from build123d import *

# Parameters (mm, degrees)
ESBO_O1_R                     = 8
RESSALTO_EXTRUS_O1_DEPTH      = 16
RESSALTO_EXTRUS_O3_START      = -2
ESBO_O3_R                     = 9.25
ESBO_O3_R_2                   = 8
RESSALTO_EXTRUS_O3_DEPTH      = 2
ESBO_O4_R                     = 7
CORTE_EXTRUS_O1_DEPTH         = 10
RESSALTO_EXTRUS_O2_DEPTH      = 4
RESSALTO_EXTRUS_O2_DEPTH_BACK = 16
ESBO_O2_R                     = 1.15
FILETE1_R                     = 1
PADR_O_LINEAR1_COUNT          = 11
PADR_O_LINEAR1_PITCH          = 0.5
CHANFRO1_SIZE                 = 0.2


with BuildPart() as part:
    # Esboço1 → Ressalto-extrusão1 (new body)
    with BuildSketch(Plane.XY):
        Circle(ESBO_O1_R)
    extrude(amount=RESSALTO_EXTRUS_O1_DEPTH)

    # Esboço3 → Ressalto-extrusão3 (add)
    with BuildSketch(Plane.XY.offset(7.5).offset(RESSALTO_EXTRUS_O3_START)):
        Circle(ESBO_O3_R)
        Circle(ESBO_O3_R_2, mode=Mode.SUBTRACT)
    extrude(amount=RESSALTO_EXTRUS_O3_DEPTH)

    # Esboço4 → Corte-extrusão1 (cut)
    with BuildSketch(Plane(origin=(0, 0, 0), x_dir=(-1, 0, 0), z_dir=(0, 0, -1))):
        Circle(ESBO_O4_R)
    extrude(amount=-CORTE_EXTRUS_O1_DEPTH, mode=Mode.SUBTRACT)

    # Esboço2 → Ressalto-extrusão2 (add, two sides: drawn at the far end of the back side and taken through both)
    with BuildSketch(Plane.XY.offset(16).offset(-RESSALTO_EXTRUS_O2_DEPTH_BACK)):
        with Locations((0, 4)):
            Circle(ESBO_O2_R)
        with Locations((3.708099244, -1.5)):
            Circle(ESBO_O2_R)
        with Locations((-3.708099244, -1.5)):
            Circle(ESBO_O2_R)
    extrude(amount=RESSALTO_EXTRUS_O2_DEPTH + RESSALTO_EXTRUS_O2_DEPTH_BACK)

    # Filete1
    filete1_edges = [part.edges().sort_by_distance(p)[0] for p in [
        (2.558099244, -1.5, 0),
        (-4.858099244, -1.5, 0),
        (-1.15, 4, 0),
    ]]
    fillet(filete1_edges, radius=FILETE1_R)

    # Esboço5 → Revolução1 (revolve)
    with BuildSketch(Plane(origin=(0, 0, 0), x_dir=(1, 0, 0), z_dir=(0, 1, 0)), mode=Mode.PRIVATE) as revolu_o1_sk:
        Polygon((8, 0), (8.433012702, -0.25), (8, -0.5), align=None)
    revolu_o1 = revolve(revolu_o1_sk.sketch.rotate(Axis((0, 0, -3.692698903), (0, 0, 1)), 180), axis=Axis((0, 0, -3.692698903), (0, 0, 1)))

    # Padrão linear1: Revolução1 ×11
    with Locations(*[(0, 0, i * PADR_O_LINEAR1_PITCH) for i in range(1, PADR_O_LINEAR1_COUNT)]):
        add(revolu_o1)

    # Chanfro1
    chanfro1_edges = [part.edges().sort_by_distance(p)[0] for p in [
        (-9.25, 0, 5.5),
    ]]
    chamfer(chanfro1_edges, length=CHANFRO1_SIZE)


solid = part.part
Design review of the part built by this model. Coordinates are the model's own, in mm. A direction names the side the tool comes from. Give positions to 0.01 mm unless a question says otherwise; leave off trailing zeros. Loops run counter-clockwise (first coordinate to the right, second up) from the corner with the lowest first, then second, coordinate; pieces in that order, holes last. Notation, with made-up numbers: (86, 12.25) -> (107, 12.25) arc R16 ccw to (107, 24.25) -> close; hole circle Ø8 at (-30, -28.75). An arc over 180 degrees is marked (long way). One line per question, with ' | ' between items. Start each with the question number.
(1) Insertion check: P1, Ø4, axis at y = 6.5, z = 12, coming from the -X side; P2, Ø4, axis at x = -2, z = 14.5, coming from the +Y side; P3, Ø8, axis at x = -6.5, y = -6.5, coming from the -Z side; P4, Ø1.5, axis at y = -7, z = 13, coming from the +X side. Each pin has a flat end and moves straight along its axis. Give the tip position at first contact, or say it passes through.
(2) We need section B-B (z = 8.75). State the section outline as (x, y) points, and give its area (3 significant figures).
(3) For line 1 (Y direction, x = 0, z = 7); line 2 (X direction, y = -0.25, z = 6.5); line 3 (Y direction, x = 3, z = 9.5), list the stretches that pass through material, from the lowest coordinate up.
(4) For faces 4 (the face through (-0.15, 5.14, 17.97)), 5 (the face through (4, -6, 0)), list the 3-axis set-ups (+Z, -Z, +X, -X, +Y, -Y) from which the entire face can be reached by the end or side of a thin tool; tool diameter is ignored.
(5) Draft analysis for pull direction X (two halves, no side actions). For faces 1 (the face through (-0.15, 5.14, 5.44)), 2 (the face through (-4, -1, 20)), 3 (the face through (-2.01, -9.03, 6.59)), state which applies: +X half, -X half, draft (parallel to the pull), parting line (faces both ways), or undercut.
(6) We need section C-C (z = 14.5). State the section outline as (x, y) points, and give its area (3 significant figures).
(7) We need section A-A (z = 6.75). State the section outline as (x, y) points, and give its area (3 significant figures).
The answers:
1) P1: stops at x = -6.61 | P2: stops at y = 8 | P3: stops at z = 0 | P4: stops at x = 4.99
2) outline: circle Ø16 at (0, 0); circle Ø2.3 at (-3.71, -1.5); circle Ø2.3 at (0, 4); circle Ø2.3 at (3.71, -1.5); hole circle Ø14 at (0, 0) | area: 59.6 mm^2
3) line 1: y = -9.25 to -7, 2.85 to 5.15, 7 to 9.25 | line 2: x = -9.25 to -7, 7 to 9.25 | line 3: y = -7.42 to -6.32, -2.41 to -0.59, 6.32 to 7.42
4) face 4: +Z | face 5: -Z, +X, -X, +Y, -Y
5) face 1: undercut | face 2: draft | face 3: parting line
6) outline: circle Ø16 at (0, 0) | area: 201 mm^2
7) outline: circle Ø18.5 at (0, 0); circle Ø2.3 at (-3.71, -1.5); circle Ø2.3 at (0, 4); circle Ø2.3 at (3.71, -1.5); hole circle Ø14 at (0, 0) | area: 127 mm^2
